```python
from build123d import *

# Parameters (mm, degrees)
BOSS_EXTRUDE1_OUTLINE_R = 50
BOSS_EXTRUDE1_DEPTH     = 0.8
SKETCH2_R               = 1.025
CUT_EXTRUDE5_DEPTH      = 10


# Read off the part's stored shape, not the designer's step: Boss-Extrude1
with BuildPart() as part:
    # Boss-Extrude1 outline → Boss-Extrude1 (new body)
    with BuildSketch(Plane.XY):
        Circle(BOSS_EXTRUDE1_OUTLINE_R)
        with BuildLine():
            ThreePointArc((-10.640683383, -13.893374577), (-6.680080661, -16.174873179), (-2.263779528, -17.352962348))
            Line((-2.263779528, -17.352962348), (-1.802339331, -24.433615634))
            ThreePointArc((-1.802339331, -24.433615634), (-9.36241701, -22.64056421), (-15.980874836, -18.570450707))
            Line((-15.980874836, -18.570450707), (-10.640683383, -13.893374577))
        make_face(mode=Mode.SUBTRACT)
        with BuildLine():
            ThreePointArc((-17.348198754, -2.3), (-16.160892844, -6.713832175), (-13.871131205, -10.669663495))
            Line((-13.871131205, -10.669663495), (-18.551621667, -16.00272894))
            ThreePointArc((-18.551621667, -16.00272894), (-22.629525039, -9.389067926), (-24.431476591, -1.831106659))
            Line((-24.431476591, -1.831106659), (-17.348198754, -2.3))
        make_face(mode=Mode.SUBTRACT)
        with BuildLine():
            ThreePointArc((2.3, -17.348198754), (6.713832175, -16.160892844), (10.669663495, -13.871131205))
            Line((10.669663495, -13.871131205), (16.00272894, -18.551621667))
            ThreePointArc((16.00272894, -18.551621667), (9.389067926, -22.629525039), (1.831106659, -24.431476591))
            Line((1.831106659, -24.431476591), (2.3, -17.348198754))
        make_face(mode=Mode.SUBTRACT)
        with BuildLine():
            ThreePointArc((13.893374577, -10.640683383), (16.174873179, -6.680080661), (17.352962348, -2.263779528))
            Line((17.352962348, -2.263779528), (24.433615634, -1.802339331))
            ThreePointArc((24.433615634, -1.802339331), (22.64056421, -9.36241701), (18.570450707, -15.980874836))
            Line((18.570450707, -15.980874836), (13.893374577, -10.640683383))
        make_face(mode=Mode.SUBTRACT)
        with BuildLine():
            ThreePointArc((-13.893374577, 10.640683383), (-16.174873179, 6.680080661), (-17.352962348, 2.263779528))
            Line((-17.352962348, 2.263779528), (-24.433615634, 1.802339331))
            ThreePointArc((-24.433615634, 1.802339331), (-22.64056421, 9.36241701), (-18.570450707, 15.980874836))
            Line((-18.570450707, 15.980874836), (-13.893374577, 10.640683383))
        make_face(mode=Mode.SUBTRACT)
        with BuildLine():
            ThreePointArc((-2.3, 17.348198754), (-6.713832175, 16.160892844), (-10.669663495, 13.871131205))
            Line((-10.669663495, 13.871131205), (-16.00272894, 18.551621667))
            ThreePointArc((-16.00272894, 18.551621667), (-9.389067926, 22.629525039), (-1.831106659, 24.431476591))
            Line((-1.831106659, 24.431476591), (-2.3, 17.348198754))
        make_face(mode=Mode.SUBTRACT)
        with BuildLine():
            ThreePointArc((-1.5, -4.769696007), (-5, 0), (-1.5, 4.769696007))
            Line((-1.5, 4.769696007), (-1.5, 7))
            Line((-1.5, 7), (1.5, 7))
            Line((1.5, 7), (1.5, 4.769696007))
            ThreePointArc((1.5, 4.769696007), (5, 0), (1.5, -4.769696007))
            Line((1.5, -4.769696007), (1.5, -7))
            Line((1.5, -7), (-1.5, -7))
            Line((-1.5, -7), (-1.5, -4.769696007))
        make_face(mode=Mode.SUBTRACT)
        with BuildLine():
            ThreePointArc((17.348198754, 2.3), (16.160892844, 6.713832175), (13.871131205, 10.669663495))
            Line((13.871131205, 10.669663495), (18.551621667, 16.00272894))
            ThreePointArc((18.551621667, 16.00272894), (22.629525039, 9.389067926), (24.431476591, 1.831106659))
            Line((24.431476591, 1.831106659), (17.348198754, 2.3))
        make_face(mode=Mode.SUBTRACT)
        with BuildLine():
            ThreePointArc((10.640683383, 13.893374577), (6.680080661, 16.174873179), (2.263779528, 17.352962348))
            Line((2.263779528, 17.352962348), (1.802339331, 24.433615634))
            ThreePointArc((1.802339331, 24.433615634), (9.36241701, 22.64056421), (15.980874836, 18.570450707))
            Line((15.980874836, 18.570450707), (10.640683383, 13.893374577))
        make_face(mode=Mode.SUBTRACT)
    extrude(amount=BOSS_EXTRUDE1_DEPTH)

    # Sketch2 → Cut-Extrude5 (cut)
    with BuildSketch(Plane.XY):
        with Locations((0, 20)):
            Circle(SKETCH2_R)
        with Locations((14.142135624, 14.142135624)):
            Circle(SKETCH2_R)
        with Locations((20, 0)):
            Circle(SKETCH2_R)
        with Locations((14.142135624, -14.142135624)):
            Circle(SKETCH2_R)
        with Locations((0, -20)):
            Circle(SKETCH2_R)
        with Locations((-14.142135624, -14.142135624)):
            Circle(SKETCH2_R)
        with Locations((-20, 0)):
            Circle(SKETCH2_R)
        with Locations((-14.142135624, 14.142135624)):
            Circle(SKETCH2_R)
    extrude(amount=CUT_EXTRUDE5_DEPTH, mode=Mode.SUBTRACT)


solid = part.part
```
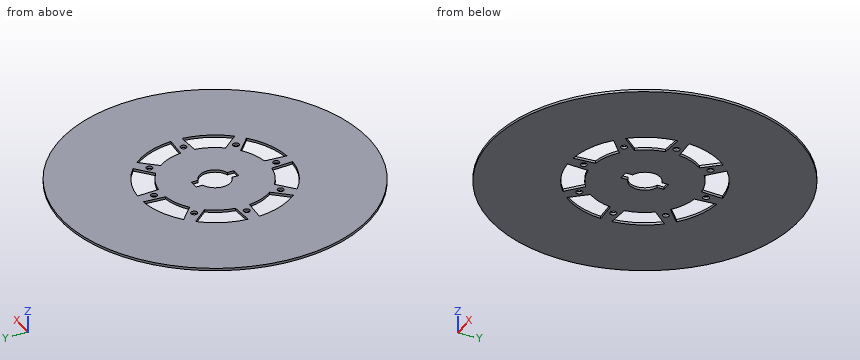
Check sheet for the modelled part. Datum: model origin and axes. Units: mm. Round coordinates to 2 decimals unless told otherwise and drop trailing zeros. Order: outer loops, then holes, each group sorted by start corner. A loop starts at its lowest first (then second) coordinate and runs counter-clockwise, first axis right, second up.
1) Scan lines: line 1 (X direction, y = 11, z = 0.3) (3 decimals); line 2 (Y direction, x = 20, z = 0.55) (3 decimals); line 3 (X direction, y = 3, z = 0.55). Record each from-to range of solid material in increasing order.
2) Section check C-C (x = 34.5). Record the boundary of the cut face in (y, z), and give its area (3 significant figures).
3) Section check A-A (z = 0.35). Give the number of separate pieces and of enclosed holes in the cut face, and give its area (3 significant figures).
4) Section check B-B (y = 33.5). Record the boundary of the cut face in (x, z), and give its area (3 significant figures).
Result:
1. line 1: x = -48.775 to -21.892, -14.208 to 14.161, 21.892 to 48.775
1. line 2: y = -45.826 to -14.151, -2.091 to -1.025, 1.025 to 2.124, 14.151 to 45.826
1. line 3: x = -49.91 to -24.32, -17.24 to -4, 4 to 17.24, 24.32 to 49.91
2. outline: (-36.19, 0) - (36.19, 0) - (36.19, 0.8) - (-36.19, 0.8) - close
2. area: 57.9 mm2
3. separate pieces: 1
3. enclosed holes: 17
3. area: 7,040 mm2
4. outline: (-37.12, 0) - (37.12, 0) - (37.12, 0.8) - (-37.12, 0.8) - close
4. area: 59.4 mm2
